Source: three-view drawing plus pictorial views. Frame: mm from the lowest corner of the part. A direction names the side the tool comes from. Coordinates: 2 decimals unless noted, no trailing zeros. Write each loop counter-clockwise with the first axis right and the second up, starting at its lowest first coordinate (ties: lowest second). Pieces come first, ordered by that corner, then holes. Notation, with made-up numbers: (75, 45) -> (92, 45) arc R8 ccw to (92, 58) -> close; hole circle Ø6 at (17, 27). An arc over 180 degrees is marked (long way). One line per question, with ' | ' between items. Start each with the question number.
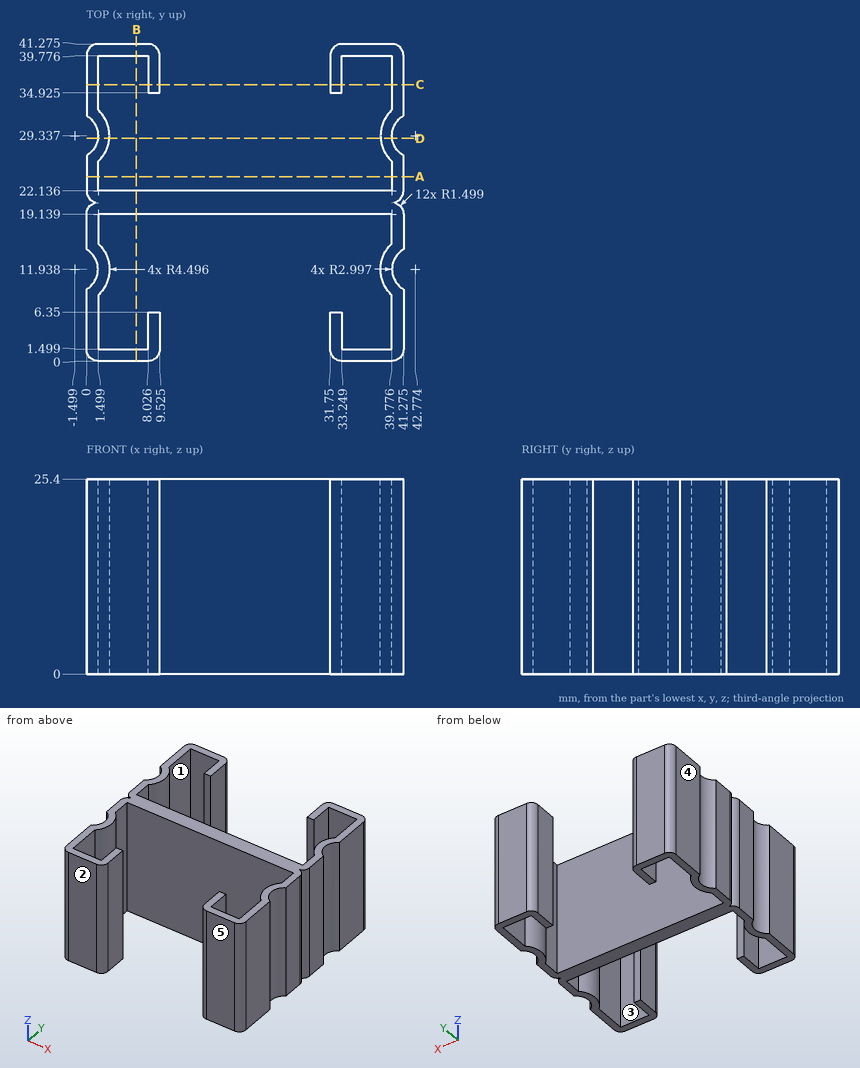
1) Section B-B, the plane x = 6.5. Return loops of the section in (y, z) (1 decimal), then the cut area to 3 significant figures.
2) Pull-direction query (X, two-part tool) for the marked faces 3, 4 and 5; classes: released by +X, released by -X, zero draft, split by the parting line, or undercut.
3) First-contact query: P1, Ø5.5, axis at y = 37, z = 14, coming from the -X side; P2, Ø10, axis at x = 19.5, z = 7.5, coming from the +Y side; P3, Ø1.5, axis at x = 14, z = 18, coming from the -Y side; P4, Ø1.2, axis at x = 32.5, z = 8, coming from the -Y side. Flat tips, straight axial feed; report the tip coordinate or a pass-through.
4) Section A-A, the plane y = 24. Return loops of the section in (x, z) (1 decimal).
5) Ray query, line 1 (Y direction, x = 34.5, z = 18) (1 decimal); line 2 (Y direction, x = 39, z = 13) (1 decimal); line 3 (X direction, y = 25.5, z = 13.5) (1 decimal). Return the intervals inside material, ascending.
6) Section D-D, the plane y = 29. Return loops of the section in (x, z) (1 decimal).
7) Section C-C, the plane y = 36. Give the number of separate pieces and of enclosed holes in the cut face, then the cut area to 3 significant figures.
8) Access query for the marked faces 1 and 2. Directions: +Z, -Z, +X, -X, +Y, -Y. A direction counts if a zero-diameter tool reaches every point of the face in a straight line with its end or side. Return the directions, or none.
Answer block:
1) outline: (0, 0) -> (1.5, 0) -> (1.5, 25.4) -> (0, 25.4) -> close; (19.1, 0) -> (22.1, 0) -> (22.1, 25.4) -> (19.1, 25.4) -> close; (39.8, 0) -> (41.3, 0) -> (41.3, 25.4) -> (39.8, 25.4) -> close | area: 152 mm2
2) face 3: undercut | face 4: released by -X | face 5: zero draft
3) P1: stops at x = 0 | P2: stops at y = 22.14 | P3: stops at y = 19.14 | P4: stops at y = 0.01
4) outline: (0, 0) -> (1.5, 0) -> (1.5, 25.4) -> (0, 25.4) -> close; (39.8, 0) -> (41.3, 0) -> (41.3, 25.4) -> (39.8, 25.4) -> close
5) line 1: y = 0 to 1.5, 19.1 to 22.1, 39.8 to 41.3 | line 2: y = 0 to 1.5, 9.5 to 14.4, 19.1 to 22.1, 26.9 to 31.8, 39.8 to 41.3 | line 3: x = 0 to 1.5, 39.8 to 41.3
6) outline: (1.5, 0) -> (3, 0) -> (3, 25.4) -> (1.5, 25.4) -> close; (38.3, 0) -> (39.8, 0) -> (39.8, 25.4) -> (38.3, 25.4) -> close
7) separate pieces: 4 | enclosed holes: 0 | area: 152 mm2
8) face 1: +Z, -Z | face 2: +Z, -Z, +X, -X, -Y
